The model under review builds one solid part; all positions refer to its coordinate system, in mm. A direction names the side the tool comes from. Give positions to 0.01 mm unless a question says otherwise; leave off trailing zeros. Write each loop counter-clockwise with the first axis right and the second up, starting at its lowest first coordinate (ties: lowest second). Pieces come first, ordered by that corner, then holes. Notation, with made-up numbers: M 40.25,44.25 L 90.25,44.25 A30 cw 90.25,76.25 Z; hole C 86,1.25 d1. An arc over 180 degrees is marked long. Write each question's results on one line, items separated by ' | '. Start each with the question number.
from build123d import *

# Parameters (mm, degrees)
SKETCH3_R           = 1.1303
BOSS_EXTRUDE1_DEPTH = 9.525
CHAMFER1_SIZE       = 0.254
CUT_EXTRUDE1_START  = 0.254
CUT_EXTRUDE1_DEPTH  = 11.051187256
FILLET1_R           = 0.127


with BuildPart() as part:
    # Sketch2 → Revolve1 (revolve)
    with BuildSketch(Plane(origin=(0, 0, 0), x_dir=(0, 0, -1), z_dir=(1, 0, 0))):
        with BuildLine():
            Line((0, 0), (2.7813, 0))
            ThreePointArc((2.7813, 0), (1.72225533, 1.469884796), (0, 2.032))
            Line((0, 2.032), (0, 0))
        make_face()
    revolve(axis=Axis((0, 0.415157056, 0), (0, -1, 0)))

    # Sketch3 → Boss-Extrude1 (add)
    with BuildSketch(Plane.XZ):
        with Locations(Location((0, 0, 0), (0, 0, 90))):
            Circle(SKETCH3_R)
    extrude(amount=BOSS_EXTRUDE1_DEPTH)

    # Chamfer1
    chamfer1_edges = [part.edges().sort_by_distance(p)[0] for p in [
        (0, -9.525, -1.1303),
    ]]
    chamfer(chamfer1_edges, length=CHAMFER1_SIZE)

    # Sketch4 → Cut-Extrude1 (cut, through all)
    with BuildSketch(Plane(origin=(0, 0, 0), x_dir=(1, 0, 0), z_dir=(0, 1, 0)).offset(CUT_EXTRUDE1_START)):
        Polygon((-0.4064, 0.4064), (-0.4064, 2.7813), (0.4064, 2.7813), (0.4064, 0.4064), (2.7813, 0.4064), (2.7813, -0.4064), (0.4064, -0.4064), (0.4064, -2.7813), (-0.4064, -2.7813), (-0.4064, -0.4064), (-2.7813, -0.4064), (-2.7813, 0.4064), align=None)
    extrude(amount=CUT_EXTRUDE1_DEPTH, mode=Mode.SUBTRACT)

    # Fillet1
    fillet1_edges = [part.edges().sort_by_distance(p)[0] for p in [
        (0.4064, 1.114434201, -0.4064),
        (-0.4064, 1.114434201, -0.4064),
        (-0.4064, 1.114434201, 0.4064),
        (0.4064, 1.114434201, 0.4064),
    ]]
    fillet(fillet1_edges, radius=FILLET1_R)


solid = part.part
(1) Add section C-C (y = 0.5). State the section outline as (x, z) points.
(2) Draft analysis for pull direction X (two halves, no side actions). For faces 5 (the flat face through (-0.406, 1, -1)), 6 (the flat face through (-0.406, 1, 1)), 7 (the cylindrical face through (-0.34, -4.57, 1.08)), 8 (the flat face through (0, -9.525, 0)), state which applies: pulls with the +X half, pulls with the -X half, needs draft (parallel to the pull), parting line crosses it, or undercut.
(3) Clearance check with flat-ended pins moving along their axes: P1, Ø3, axis at x = 0, y = -5.5, coming from the +Z side; P2, Ø2, axis at x = -1.5, z = -2, coming from the -Y side; P3, Ø0.5, axis at x = -2, y = 1, coming from the +Z side; P4, Ø1.5, axis at x = 0.5, z = -1, coming from the -Y side (3 decimals). State where each tip first meets the part, or that it passes through.
(4) Add section B-B (x = 0). State the section outline as (y, z) points (3 decimals).
(5) Machinability: for faces 1 (the flat face through (0, 0.254, 0)), 2 (the flat face through (-1, 0, 1)), 3 (the flat face through (1, 1, 0.406)), 4 (the flat face through (0.406, 1, 1)), which of the approach directions +Z, -Z, +X, -X, +Y, -Y give a long, thin tool a straight path to every point of the face, cutting with its end or side? Answer none if there is none.
(6) Wall thickness on L1, parallel to X at y = 0.75, z = 0.75; L2, parallel to Y at x = 0.3, z = 0 (3 decimals); L3, parallel to Z at x = 1.3, y = 0.75: over which ranges is each line inside the solid? List them lowest first.
(7) Add section A-A (z = 0). State the section outline as (x, y) points (3 decimals), then the cut area to 3 significant figures.
Calculated:
1) outline: M -2.54,-0.41 A2.57 ccw -0.41,-2.54 L -0.41,-0.53 A0.13 ccw -0.53,-0.41 Z; M -2.54,0.41 L -0.53,0.41 A0.13 ccw -0.41,0.53 L -0.41,2.54 A2.57 ccw Z; M 0.41,-2.54 A2.57 ccw 2.54,-0.41 L 0.53,-0.41 A0.13 ccw 0.41,-0.53 Z; M 0.41,0.53 A0.13 ccw 0.53,0.41 L 2.54,0.41 A2.57 ccw 0.41,2.54 Z
2) face 5: undercut | face 6: undercut | face 7: parting line crosses it | face 8: needs draft
3) P1: stops at z = 1.13 | P2: stops at y = 0 | P3: stops at z = 1.51 | P4: stops at y = -9.525
4) outline: M -9.525,-0.876 L -9.271,-1.13 L 0,-1.13 L 0,-2.781 A2.919 ccw 0.254,-2.687 L 0.254,2.687 A2.919 ccw 0,2.781 L 0,1.13 L -9.271,1.13 L -9.525,0.876 Z
5) face 1: +Y | face 2: -Y | face 3: +X, -X, +Y | face 4: +Z, -Z, +Y
6) L1: x = -2.3 to -0.41, 0.41 to 2.3 | L2: y = -9.525 to 0.254 | L3: z = -2.04 to -0.41, 0.41 to 2.04
7) outline: M -2.781,0 L -1.13,0 L -1.13,-9.271 L -0.876,-9.525 L 0.876,-9.525 L 1.13,-9.271 L 1.13,0 L 2.781,0 A2.919 ccw 2.687,0.254 L -2.687,0.254 A2.919 ccw Z | area: 22.9 mm²
